Read the model definition and answer for the solid it produces. Units are mm, in the model's axes. Face numbers are marked on the shaded views. A direction names the side the tool comes from. Give positions to 0.01 mm unless a question says otherwise; leave off trailing zeros. Loops run counter-clockwise (first coordinate to the right, second up) from the corner with the lowest first, then second, coordinate; pieces in that order, holes last. Notation, with made-up numbers: (74.5, 6) -> (87.5, 6) arc R15 cw to (87.5, 23) -> close; hole circle Ø3 at (81, -25). An arc over 180 degrees is marked (long way). Answer as CSV lines item,"result". Start each with the question number.
```python
from build123d import *

# Parameters (mm, degrees)
CUT_EXTRUDE1_DEPTH  = 1.349999904
CIRPATTERN1_COUNT   = 24
SKETCH17_R          = 31.75
BOSS_EXTRUDE1_DEPTH = 2.1
SKETCH15_W          = 26.9875
SKETCH15_H          = 26.9875
CUT_EXTRUDE2_DEPTH  = 9.45
SKETCH16_W          = 30.1625
SKETCH16_H          = 30.1625
CUT_EXTRUDE3_DEPTH  = 1.5875


with BuildPart() as part:
    # Sketch2 → Revolve1 (revolve)
    with BuildSketch(Plane.XY):
        Polygon((0, 0), (31.75, 0), (31.75, 1.5875), (22.225, 5.55625), (22.225, 6.35), (0, 6.35), align=None)
    revolve(axis=Axis((0, 6.35, 0), (0, -1, 0)))

    # Sketch3 → Cut-Extrude1 (cut, symmetric)
    with BuildSketch(Plane.XY):
        Polygon((22.225, 6.35), (31.75, 2.38125), (31.75, 0), (22.225, 0), align=None)
    cut_extrude1 = extrude(amount=CUT_EXTRUDE1_DEPTH, both=True, mode=Mode.SUBTRACT)

    # CirPattern1: Cut-Extrude1 ×24 about axis
    cirpattern1_axis = Axis((0, 0, 0), (0, 1, 0))
    for i in range(1, CIRPATTERN1_COUNT):
        add(cut_extrude1.rotate(cirpattern1_axis, i * 360 / CIRPATTERN1_COUNT), mode=Mode.SUBTRACT)

    # Sketch17 → Boss-Extrude1 (add)
    with BuildSketch(Plane.XZ):
        Circle(SKETCH17_R)
    extrude(amount=BOSS_EXTRUDE1_DEPTH)

    # Sketch15 → Cut-Extrude2 (cut, through all)
    with BuildSketch(Plane(origin=(0, 6.35, 0), x_dir=(1, 0, 0), z_dir=(0, 1, 0))):
        Rectangle(SKETCH15_W, SKETCH15_H)
    extrude(amount=-CUT_EXTRUDE2_DEPTH, mode=Mode.SUBTRACT)

    # Sketch16 → Cut-Extrude3 (cut)
    with BuildSketch(Plane(origin=(0, 6.35, 0), x_dir=(1, 0, 0), z_dir=(0, 1, 0))):
        Rectangle(SKETCH16_W, SKETCH16_H)
    extrude(amount=-CUT_EXTRUDE3_DEPTH, mode=Mode.SUBTRACT)


solid = part.part
```
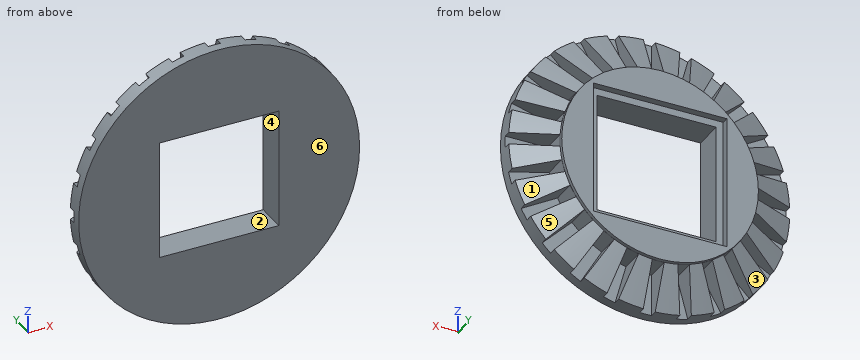
(1) Find section A-A on y = -1. Write down the section's boundary in (x, z), then the cut area to 3 significant figures.
(2) The mould has two halves that part along X. Classify the marked faces 3, 4, 5 and 6: pulls with the +X half, pulls with the -X half, needs draft (parallel to the pull), parting line crosses it, or undercut.
(3) A tool of negligible diameter and unlimited length cuts with its end or side. For the marked faces 1 and 2, from which of +Z, -Z, +X, -X, +Y, -Y can it reach the whole face along a straight path? Write none if from no direction.
(4) Each of these flat-tipped pins is pushed along its axis until it touches: P1, Ø3, axis at y = 1.5, z = -26.5, coming from the -X side; P2, Ø7, axis at x = 17, z = 19.5, coming from the +Y side; P3, Ø4, axis at y = 2.5, z = -20.5, coming from the +X side. Where does it stop, or does it pass through?
(5) Find the intervals of material crossed by line 1 along X through (y, z) = (0.5, -20.5); line 2 along X through (y, z) = (1.75, -7); line 3 along X through (y, z) = (1, -13), in increasing order. Write a range as from..to.
Answer block:
1,outline,"circle Ø63.5 at (0, 0); hole (-13.49, -13.49) -> (13.49, -13.49) -> (13.49, 13.49) -> (-13.49, 13.49) -> close"
1,area,"2,440 mm2"
2,face 3,"pulls with the -X half"
2,face 4,"undercut"
2,face 5,"pulls with the +X half"
2,face 6,"needs draft"
3,face 1,"-Z, +X, +Y"
3,face 2,"+Y, -Y"
4,P1,"stops at x = -19.57"
4,P2,"stops at y = 5.5"
4,P3,"stops at x = 25.64"
5,line 1,"x = -24.24..-22.41, -18.59..-13.39, -10.28..10.28, 13.39..18.59, 22.41..24.24"
5,line 2,"x = -21.13..-13.49, 13.49..21.13"
5,line 3,"x = -28.97..-25.22, -19.82..-13.49, 13.49..19.82, 25.22..28.97"
